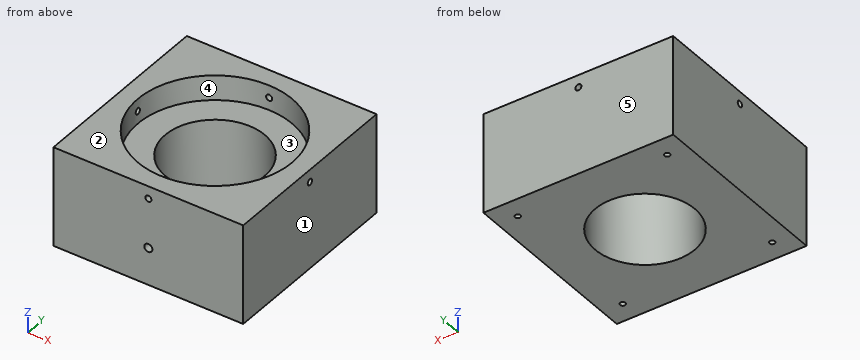
Autodesk Inventor part; units mm, degrees
ref_plane "YZ Plane" through (0, 0, 0) normal (1, 0, 0) x (0, 1, 0)
ref_plane "XZ Plane" through (0, 0, 0) normal (0, 1, 0) x (-1, 0, 0)
ref_plane "XY Plane" through (0, 0, 0) normal (0, 0, 1) x (1, 0, 0)
sketch "Sketch1" plane through (0, 0, 0) normal (0, 0, 1) x (1, 0, 0)
  line L0 (-38.1, 38.1) -> (38.1, 38.1)
  line L1 (38.1, 38.1) -> (38.1, -38.1)
  line L2 (38.1, -38.1) -> (-38.1, -38.1)
  line L3 (-38.1, -38.1) -> (-38.1, 38.1)
  point P0 (0, 0)
  dimension "d0" = 76.2
  dimension "d1" = 76.2
  dimension "d2" = 38.1
  dimension "d3" = 38.1
extrude "baseExtrusion" add sketch "Sketch1" along normal blind 40
sketch "Sketch2" plane through (0, 0, 40) normal (0, 0, 1) x (1, 0, 0)
  circle A0 centre (0, 0) radius 31
  dimension "d6" = 62
extrude "tlExtrusion" cut sketch "Sketch2" against normal blind 10
sketch "Sketch3" plane through (0, 0, 0) normal (0, 0, -1) x (-1, 0, 0)
  circle A0 centre (0, 0) radius 20
  dimension "d9" = 40
extrude "lightPathExtrusion" cut sketch "Sketch3" against normal through all
sketch "Sketch4" plane through (38.1, -38.1, 0) normal (1, 0, 0) x (0, 0, -1)
  line L0 (0, 76.2) -> (0, 0)
  line L1 (-40, 0) -> (-40, 76.2)
  point P0 (0, 38.1)
  point P1 (-35, 38.1)
  point P2 (0, 38.1)
  dimension "d12" = 5
hole "tubeLensGrubScrew1" at (38.1, 0, 35) direction (-1, 0, 0) diameter 2.459 end through all
pattern_circular "tubeLensGrubScrew2" count 2 over 90 about axis through (0, 0, -10) along (0, 0, 1) of "tubeLensGrubScrew1"
sketch "Sketch5" plane through (0, 0, 0) normal (0, 0, -1) x (-1, 0, 0)
  point P0 (0, 0)
  point P1 (-30, -30)
  point P2 (-30, 30)
  point P3 (30, -30)
  point P4 (30, 30)
  dimension "d23" = 60
  dimension "d24" = 60
  dimension "d25" = 30
  dimension "d26" = 30
hole "60mmCageSystem" at (30, -30, 0) at (30, 30, 0) at (-30, -30, 0) at (-30, 30, 0) direction (0, 0, 1) diameter 2.156 depth 10 tip angle 118
sketch "Sketch6" plane through (-38.1, -38.1, 0) normal (0, -1, 0) x (1, 0, 0)
  line L0 (76.2, 0) -> (0, 0)
  point P0 (38.1, 0)
  point P1 (38.1, 15)
  point P2 (38.1, 0)
  dimension "d34" = 15
hole "m6MountingHole" at (0, -38.1, 15) direction (0, 1, 0) diameter 3.242 depth 11.8 tip angle 118
properties part number "tubeLensHolder_v5"
Part model, mm, in its own coordinate system. Face numbers are marked on the shaded views. A direction names the side the tool comes from. Give positions to 0.01 mm unless a question says otherwise; leave off trailing zeros. Order: outer loops, then holes, each group sorted by start corner. A loop starts at its lowest first (then second) coordinate and runs counter-clockwise, first axis right, second up. Notation, with made-up numbers: (20.25, 39.25) - (78.25, 39.25) arc R36 cw to (78.25, 74.25) - close; hole circle Ø8 at (81, 74). An arc over 180 degrees is marked (long way). One line per question, with ' | ' between items.
1. Which spindle directions (+Z, -Z, +X, -X, +Y, -Y) get a long thin tool onto all of the face, cutting with end or side? Do the marked faces 4 and 5. Say none if no direction does.
Filled in:
face 4: +Z | face 5: +Z, -Z, +X, -X, +Y
2. Band-saw the part on B-B on x = 4.5. List the corners of the cut face in (y, z), then the cut area to 3 significant figures.
Filled in:
outline: (-38.1, 0) - (-19.49, 0) - (-19.49, 30) - (-30.67, 30) - (-30.67, 40) - (-38.1, 40) - close; (19.49, 0) - (38.1, 0) - (38.1, 40) - (30.67, 40) - (30.67, 30) - (19.49, 30) - close | area: 1,270 mm²
3. Band-saw the part on D-D on y = 14. List the corners of the cut face in (x, z), then the cut area to 3 significant figures.
Filled in:
outline: (-38.1, 0) - (-14.28, 0) - (-14.28, 30) - (-27.66, 30) - (-27.66, 40) - (-38.1, 40) - close; (14.28, 0) - (38.1, 0) - (38.1, 40) - (27.66, 40) - (27.66, 30) - (14.28, 30) - close | area: 1,640 mm²
4. Drop a flat-ended pin along its axis: P1, Ø1.7, axis at x = -30, y = -30, coming from the -Z side. Give the stop position or say it passes through.
Filled in:
P1: z = 10.14
5. Drill centre lines: probe 1 along Y at (x, z) = (30, 6); probe 2 along X at (y, z) = (-34, 35). Where is each one in solid material? Low to high.
Filled in:
probe 1: -38.1 to -31.08, -28.92 to 28.92, 31.08 to 38.1 | probe 2: -38.1 to -1.23, 1.23 to 38.1
6. Band-saw the part on C-C on z = 35. List the corners of the cut face in (x, y), then the cut area to 3 significant figures.
Filled in:
outline: (-38.1, -38.1) - (-1.23, -38.1) - (-1.23, -30.98) arc R31 cw to (-30.98, -1.23) - (-38.1, -1.23) - close; (-38.1, 1.23) - (-30.98, 1.23) arc R31 cw to (-1.23, 30.98) - (-1.23, 38.1) - (-38.1, 38.1) - close; (1.23, -38.1) - (38.1, -38.1) - (38.1, -1.23) - (30.98, -1.23) arc R31 cw to (1.23, -30.98) - close; (1.23, 30.98) arc R31 cw to (30.98, 1.23) - (38.1, 1.23) - (38.1, 38.1) - (1.23, 38.1) - close | area: 2,720 mm²
7. Band-saw the part on A-A on z = 7. List the corners of the cut face in (x, y).
Filled in:
outline: (-38.1, -38.1) - (38.1, -38.1) - (38.1, 38.1) - (-38.1, 38.1) - close; hole circle Ø2.16 at (-30, -30); hole circle Ø2.16 at (-30, 30); hole circle Ø40 at (0, 0); hole circle Ø2.16 at (30, -30); hole circle Ø2.16 at (30, 30)
8. Pull direction X, two halves, no side cores. Call the marked faces 1, 2 and 3: +X half, -X half, draft (parallel to the pull), parting line (faces both ways), or undercut.
Filled in:
face 1: +X half | face 2: draft | face 3: undercut
